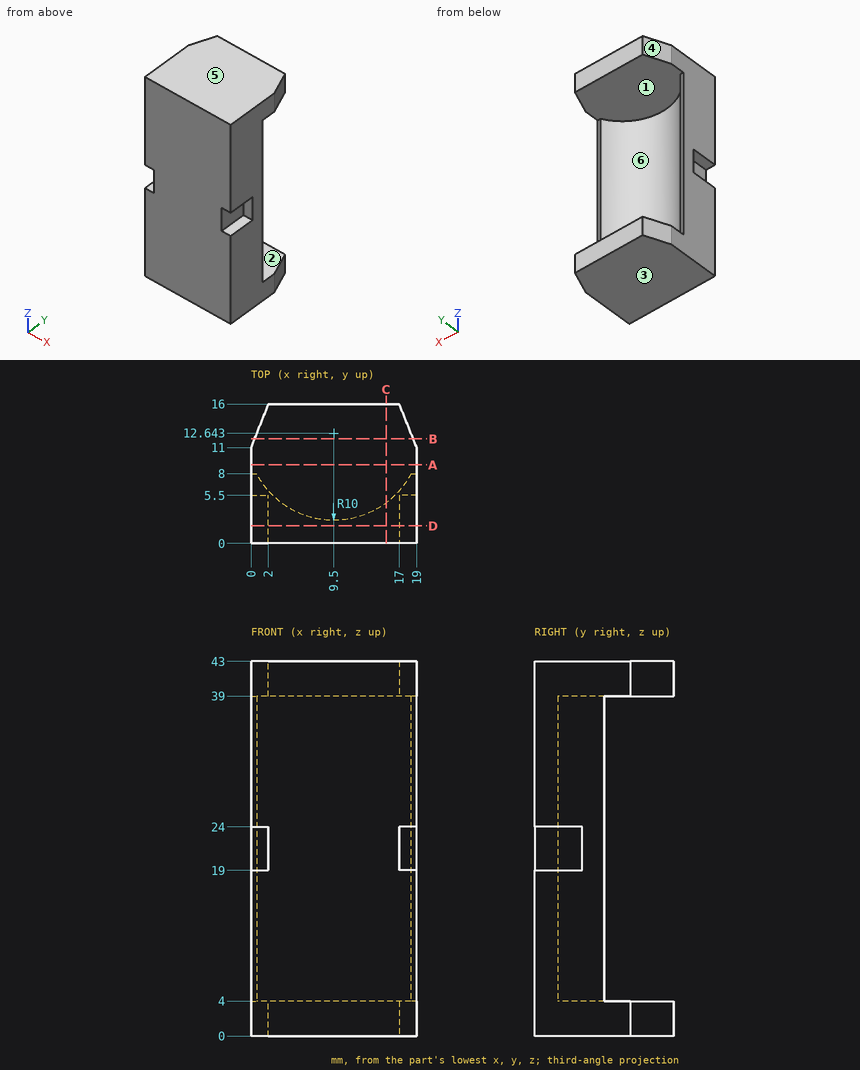
Could you check a few things on this drawing? It's one solid part, dimensions in mm from its lowest x, y, z. A direction names the side the tool comes from. Give positions to 0.01 mm unless a question says otherwise; leave off trailing zeros. Order: outer loops, then holes, each group sorted by start corner. A loop starts at its lowest first (then second) coordinate and runs counter-clockwise, first axis right, second up. Notation, with made-up numbers: (75, -14) -> (125, -14) arc R30 cw to (125, 10) -> close; hole circle Ø9 at (20, 20.5). An arc over 180 degrees is marked (long way). Answer in a Markdown table with one row per item. Add a question column.
Item 1: For the marked faces 5 and 6, which set-ups out of +Z, -Z, +X, -X, +Y, -Y let a thin tool reach every point of the face, with its end or its side?
Item 2: Imagine slicing it at D-D (y = 2). List the corners of the cut face in (x, z) for me.
Item 3: Imagine slicing it at B-B (y = 12). List the corners of the cut face in (x, z) for me, and give its area (3 significant figures).
Item 4: I'm going to push flat-ended pins straight in: P1, Ø6, axis at x = 4, z = 21.5, coming from the +Y side (1 decimal); P2, Ø4, axis at y = 11, z = 21, coming from the +X side; P3, Ø1.5, axis at y = 3.5, z = 22, coming from the +X side; P4, Ø2.5, axis at y = 1.5, z = 21, coming from the -X side. Where does each tip first touch, or does it pass through?
Item 5: Please list where these lines run through material, in increasing order: probe 1 along Z at (x, y) = (12.75, 5); probe 2 along Z at (x, y) = (1.25, 1.5); probe 3 along X at (y, z) = (6.5, 26.5).
Item 6: Imagine slicing it at C-C (x = 15.5). List the corners of the cut face in (y, z) for me.
Item 7: We'd pull the mould along Z, two halves only. Please class the marked faces 1, 2, 3 and 4: pulls with the +Z half, pulls with the -Z half, needs draft (parallel to the pull), parting line crosses it, or undercut.
Item 8: Imagine slicing it at A-A (y = 9). List the corners of the cut face in (x, z) for me, and give its area (3 significant figures).
Result:
| question | item | result |
|---|---|---|
| 1 | face 5 | +Z, +X, -X, +Y, -Y |
| 1 | face 6 | +Y |
| 2 | outline | (0, 0) -> (19, 0) -> (19, 19) -> (17, 19) -> (17, 24) -> (19, 24) -> (19, 43) -> (0, 43) -> (0, 24) -> (2, 24) -> (2, 19) -> (0, 19) -> close |
| 3 | outline | (0.4, 0) -> (18.6, 0) -> (18.6, 4) -> (0.4, 4) -> close; (0.4, 39) -> (18.6, 39) -> (18.6, 43) -> (0.4, 43) -> close |
| 3 | area | 146 mm2 |
| 4 | P1 | y = 7.4 |
| 4 | P2 | through |
| 4 | P3 | x = 17 |
| 4 | P4 | x = 2 |
| 5 | probe 1 | 0 to 4, 39 to 43 |
| 5 | probe 2 | 0 to 19, 24 to 43 |
| 5 | probe 3 | 0 to 1.61, 17.39 to 19 |
| 6 | outline | (0, 0) -> (16, 0) -> (16, 4) -> (4.64, 4) -> (4.64, 39) -> (16, 39) -> (16, 43) -> (0, 43) -> close |
| 7 | face 1 | undercut |
| 7 | face 2 | undercut |
| 7 | face 3 | pulls with the -Z half |
| 7 | face 4 | needs draft |
| 8 | outline | (0, 0) -> (19, 0) -> (19, 4) -> (0, 4) -> close; (0, 39) -> (19, 39) -> (19, 43) -> (0, 43) -> close |
| 8 | area | 152 mm2 |
